```python
from build123d import *

# Parameters (mm, degrees)
BOSS_EXTRU_1_DEPTH      = 6.5
BOSS_EXTRU_1_DEPTH_BACK = 6.5
ESQUISSE1_R             = 30
ESQUISSE1_R_2           = 6
ENL_V_MAT_EXTRU_1_DEPTH = 3.75


with BuildPart() as part:
    # Esquisse1 → Boss.-Extru.1 (new, two sides: drawn at the far end of the back side and taken through both)
    with BuildSketch(Plane.XY.offset(-BOSS_EXTRU_1_DEPTH_BACK)):
        Circle(ESQUISSE1_R)
        Circle(ESQUISSE1_R_2, mode=Mode.SUBTRACT)
    extrude(amount=BOSS_EXTRU_1_DEPTH + BOSS_EXTRU_1_DEPTH_BACK)

    # Esquisse3 → Enl_v. mat.-Extru.1 (cut)
    with BuildSketch(Plane.XY.offset(6.5)):
        with BuildLine():
            Line((-10.706656289, -13.204829083), (-24.283177855, -17.616108346))
            ThreePointArc((-24.283177855, -17.616108346), (-17.633557569, -24.270509831), (-9.25, -28.538351389))
            Line((-9.25, -28.538351389), (-9.25, -14.263151826))
            ThreePointArc((-9.25, -14.263151826), (0, -17), (9.25, -14.263151826))
            Line((9.25, -14.263151826), (9.25, -28.538351389))
            ThreePointArc((9.25, -28.538351389), (17.633557569, -24.270509831), (24.283177855, -17.616108346))
            Line((24.283177855, -17.616108346), (10.706656289, -13.204829083))
            ThreePointArc((10.706656289, -13.204829083), (16.167960777, -5.253288904), (16.423470685, 4.389716468))
            Line((16.423470685, 4.389716468), (30, 0))
            ThreePointArc((30, 0), (28.528362011, 9.280762952), (24.257829269, 17.650997681))
            Line((24.257829269, 17.650997681), (15.867077492, 6.102118637))
            ThreePointArc((15.867077492, 6.102118637), (9.992349289, 13.753288904), (0.900263096, 16.976145804))
            Line((0.900263096, 16.976145804), (9.291014873, 28.525024849))
            ThreePointArc((9.291014873, 28.525024849), (0, 30), (-9.291014873, 28.525024849))
            Line((-9.291014873, 28.525024849), (-0.900263096, 16.976145804))
            ThreePointArc((-0.900263096, 16.976145804), (-9.992349289, 13.753288904), (-15.867077492, 6.102118637))
            Line((-15.867077492, 6.102118637), (-24.257829269, 17.650997681))
            ThreePointArc((-24.257829269, 17.650997681), (-28.528362011, 9.280762952), (-30, 0))
            Line((-30, 0), (-16.423470685, 4.389716468))
            ThreePointArc((-16.423470685, 4.389716468), (-16.167960777, -5.253288904), (-10.706656289, -13.204829083))
        make_face()
    enl_v_mat_extru_1 = extrude(amount=-ENL_V_MAT_EXTRU_1_DEPTH, mode=Mode.SUBTRACT)

    # Sym_trie1: Enl_v. mat.-Extru.1 across plane
    add(enl_v_mat_extru_1.mirror(Plane.XY), mode=Mode.SUBTRACT)


solid = part.part
```
Model file for the job. Use its own axes, mm. A direction names the side the tool comes from. Round coordinates to 2 decimals unless told otherwise and drop trailing zeros. Loops run counter-clockwise (first coordinate to the right, second up) from the corner with the lowest first, then second, coordinate; pieces in that order, holes last. Notation, with made-up numbers: M 74.5,-14.75 L 128.5,-14.75 A21 cw 128.5,-2.75 Z; hole C 85,34.25 d11. An arc over 180 degrees is marked long. Put each result on its own line as item: value. Start each with the question number.
Item 1: Cut at C-C (y = 20). List the corners of the cut face in (x, z).
Item 2: Cut at A-A (x = 0). List the corners of the cut face in (y, z).
Item 3: Cut at D-D (x = 7). List the corners of the cut face in (y, z).
Item 4: Cut at B-B (z = 5.75). List the corners of the cut face in (x, y), then the cut area to 3 significant figures.
Item 5: Mould opens along X. For faces 1 (the face through (23.117, 2.226, -4.651)), 2 (the face through (0, 8, 2.75)), 3 (the face through (-23, -6, 6.5)) say: released by +X, released by -X, zero draft, split by the parting line, or undercut.
Item 6: Drill centre lines: line 1 along X through (y, z) = (0, -1.2); line 2 along Z through (x, y) = (8, 3.5). Where is each one in solid material? Low to high.
Item 7: 3-axis set-ups, long thin cutter, end or side, ignore diameter. For faces 4 (the face through (-16.21, -5.12, 4.65)), 5 (the face through (16.125, -5.383, -4.651)), 6 (the face through (-20.004, 11.796, -4.651)): which of +Z, -Z, +X, -X, +Y, -Y reach the whole face in a straight line?
Item 8: Drop flat-ended pins along their axis: P1, Ø4, axis at y = -22.5, z = 5, coming from the -X side; P2, Ø4, axis at y = 4, z = -2.5, coming from the -X side; P3, Ø1, axis at x = -15.5, z = 1, coming from the -Y side. Give the stop position or say it passes through.
Answer block:
1. outline: M -22.36,-6.5 L -3.1,-6.5 L -3.1,-2.75 L 3.1,-2.75 L 3.1,-6.5 L 22.36,-6.5 L 22.36,6.5 L 3.1,6.5 L 3.1,2.75 L -3.1,2.75 L -3.1,6.5 L -22.36,6.5 Z
2. outline: M -30,-6.5 L -17,-6.5 L -17,-2.75 L -6,-2.75 L -6,2.75 L -17,2.75 L -17,6.5 L -30,6.5 Z; M 6,-2.75 L 30,-2.75 L 30,2.75 L 6,2.75 Z
3. outline: M -29.17,-6.5 L -15.49,-6.5 L -15.49,-2.75 L 15.49,-2.75 L 15.49,-6.5 L 25.37,-6.5 L 25.37,-2.75 L 29.17,-2.75 L 29.17,2.75 L 25.37,2.75 L 25.37,6.5 L 15.49,6.5 L 15.49,2.75 L -15.49,2.75 L -15.49,6.5 L -29.17,6.5 Z
4. outline: M -30,0 A30 ccw -24.28,-17.62 L -10.71,-13.2 A17 cw -16.42,4.39 Z; M -24.26,17.65 L -15.87,6.1 A17 cw -0.9,16.98 L -9.29,28.53 A30 ccw Z; M -9.25,-28.54 A30 ccw 9.25,-28.54 L 9.25,-14.26 A17 cw -9.25,-14.26 Z; M 0.9,16.98 A17 cw 15.87,6.1 L 24.26,17.65 A30 ccw 9.29,28.53 Z; M 10.71,-13.2 L 24.28,-17.62 A30 ccw 30,0 L 16.42,4.39 A17 cw Z
4. area: 1,240 mm2
5. face 1: released by +X
5. face 2: undercut
5. face 3: zero draft
6. line 1: -30 to -6, 6 to 30
6. line 2: -2.75 to 2.75
7. face 4: +Z
7. face 5: -Z
7. face 6: -Z, -X
8. P1: x = -9.25
8. P2: x = -29.93
8. P3: y = -25.98
